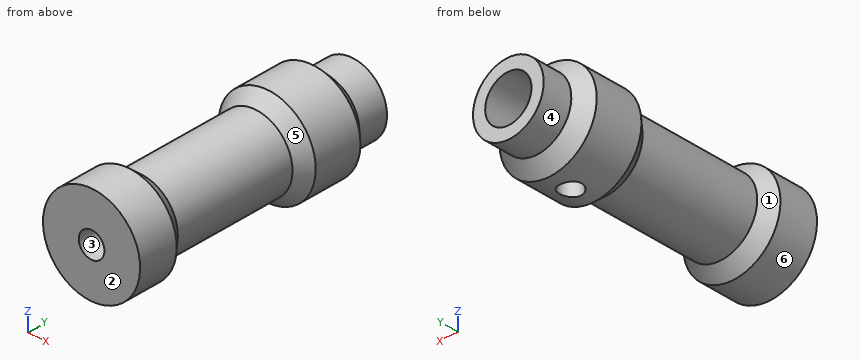
from build123d import *

# Parameters (mm, degrees)
FORO_FILETTATO_M3_5X0_6_1_D    = 2.9
FORO_FILETTATO_M3X0_5_2_REACH  = 36.283
FORO_FILETTATO_M3X0_5_2_BORE_R = 1.25


with BuildPart() as part:
    # Schizzo1 → Rivoluzione1 (revolve)
    with BuildSketch(Plane.XY, mode=Mode.PRIVATE) as rivoluzione1_sk:
        Polygon((0, 0), (5.49, 0), (5.49, 4.5), (4.24, 6), (4.24, 20.11), (5.49, 21.61), (5.49, 27.11), (3.995, 28.61), (3.995, 32.01), (2.615, 32.01), (2.615, 7.08), (0, 7.08), align=None)
    revolve(rivoluzione1_sk.sketch.rotate(Axis((0, 0, 0), (0, 1, 0)), 90), axis=Axis((0, 0, 0), (0, 1, 0)))

    # Foro filettato M3.5x0.6-1 (through all)
    with Locations(Plane(origin=(0, 0, 0), x_dir=(-1, 0, 0), z_dir=(0, -1, 0))):
        with Locations((0, 0)):
            Hole(FORO_FILETTATO_M3_5X0_6_1_D / 2)

    # Foro filettato M3x0.5-2 bore → Foro filettato M3x0.5-2 (cut, up to next)
    with BuildSketch(Plane(origin=(0, 0, -5.49), x_dir=(-1, 0, 0), z_dir=(0, 0, -1)), mode=Mode.PRIVATE) as foro_filettato_m3x0_5_2_sk1:
        with Locations((0, 24.36)):
            Circle(FORO_FILETTATO_M3X0_5_2_BORE_R)
    foro_filettato_m3x0_5_2_tool1 = extrude(foro_filettato_m3x0_5_2_sk1.sketch, amount=-FORO_FILETTATO_M3X0_5_2_REACH, mode=Mode.PRIVATE) & part.part
    add(foro_filettato_m3x0_5_2_tool1.solids().sort_by_distance((0, 24.36, -5.49))[0], mode=Mode.SUBTRACT)


solid = part.part
Design review of the part built by this model. Coordinates are the model's own, in mm. Face numbers are marked on the shaded views. A direction names the side the tool comes from. Round coordinates to 2 decimals unless told otherwise and drop trailing zeros. Loops run counter-clockwise (first coordinate to the right, second up) from the corner with the lowest first, then second, coordinate; pieces in that order, holes last. Notation, with made-up numbers: M 78,18 L 137,18 A29 cw 137,46 Z; hole C -29.5,43.25 d9. An arc over 180 degrees is marked long. Answer as a JSON object with one key per item and string values.
Item 1: Clearance check with flat-ended pins moving along their axes: P1, Ø1, axis at x = -3.5, y = 16.5, coming from the -Z side; P2, Ø1.5, axis at x = 0, y = 24.36, coming from the -Z side; P3, Ø5, axis at y = 20, z = -3, coming from the +X side. State where each tip first meets the part, or that it passes through.
Answer sheet:
{"P1": "stops at z = -3", "P2": "stops at z = 2.51", "P3": "stops at x = 5.38"}
Item 2: The part is to be moulded in two halves that separate along X. For the marked faces 1, 2 and 3, say which applies: pulls with the +X half, pulls with the -X half, needs draft (parallel to the pull), parting line crosses it, or undercut.
Answer sheet:
{"face 1": "parting line crosses it", "face 2": "needs draft", "face 3": "undercut"}
Item 3: We need section D-D on y = 30.5. Give the boundary of the cut face in (x, z) (3 decimals).
Answer sheet:
{"outline": "C 0,0 d7.99; hole C 0,0 d5.23"}
Item 4: We need section A-A on x = 0. Give the boundary of the cut face in (y, z) (3 decimals), and give its area (3 significant figures).
Answer sheet:
{"outline": "M 0,-5.49 L 4.5,-5.49 L 6,-4.24 L 20.11,-4.24 L 21.61,-5.49 L 23.11,-5.49 L 23.11,-2.615 L 7.08,-2.615 L 7.08,-1.45 L 0,-1.45 Z; M 0,1.45 L 7.08,1.45 L 7.08,2.615 L 32.01,2.615 L 32.01,3.995 L 28.61,3.995 L 27.11,5.49 L 21.61,5.49 L 20.11,4.24 L 6,4.24 L 4.5,5.49 L 0,5.49 Z; M 25.61,-5.49 L 27.11,-5.49 L 28.61,-3.995 L 32.01,-3.995 L 32.01,-2.615 L 25.61,-2.615 Z", "area": "142 mm^2"}
Item 5: We need section C-C on y = 16.5. Give the boundary of the cut face in (x, z) (3 decimals), and give its area (3 significant figures).
Answer sheet:
{"outline": "C 0,0 d8.48; hole C 0,0 d5.23", "area": "35.0 mm^2"}
Item 6: Machinability: for the marked faces 4, 5 and 6, which of the approach directions +Z, -Z, +X, -X, +Y, -Y give a long, thin tool a straight path to every point of the face, cutting with its end or side? Answer none if there is none.
Answer sheet:
{"face 4": "+Y", "face 5": "none", "face 6": "+Y, -Y"}
Item 7: We need section B-B on z = 0. Give the boundary of the cut face in (x, y) (3 decimals).
Answer sheet:
{"outline": "M -5.49,0 L -1.45,0 L -1.45,7.08 L -2.615,7.08 L -2.615,32.01 L -3.995,32.01 L -3.995,28.61 L -5.49,27.11 L -5.49,21.61 L -4.24,20.11 L -4.24,6 L -5.49,4.5 Z; M 1.45,0 L 5.49,0 L 5.49,4.5 L 4.24,6 L 4.24,20.11 L 5.49,21.61 L 5.49,27.11 L 3.995,28.61 L 3.995,32.01 L 2.615,32.01 L 2.615,7.08 L 1.45,7.08 Z"}
Item 8: Wall thickness on L1, parallel to X at y = 26.75, z = 0 (3 decimals); L2, parallel to Y at x = 1, z = 2; L3, parallel to Y at x = -1, z = -3.75: over which ranges is each line inside the solid? List them lowest first. Write a range as from..to.
Answer sheet:
{"L1": "x = -5.49..-2.615, 2.615..5.49", "L2": "y = 0..7.08", "L3": "y = 0..23.61, 25.11..32.01"}
